Design review of the part shown in the three views and the two pictorial views. Dimensions are in mm from the part's minimum x, y and z. A direction names the side the tool comes from. Give positions to 0.01 mm unless a question says otherwise; leave off trailing zeros. Loops run counter-clockwise (first coordinate to the right, second up) from the corner with the lowest first, then second, coordinate; pieces in that order, holes last.
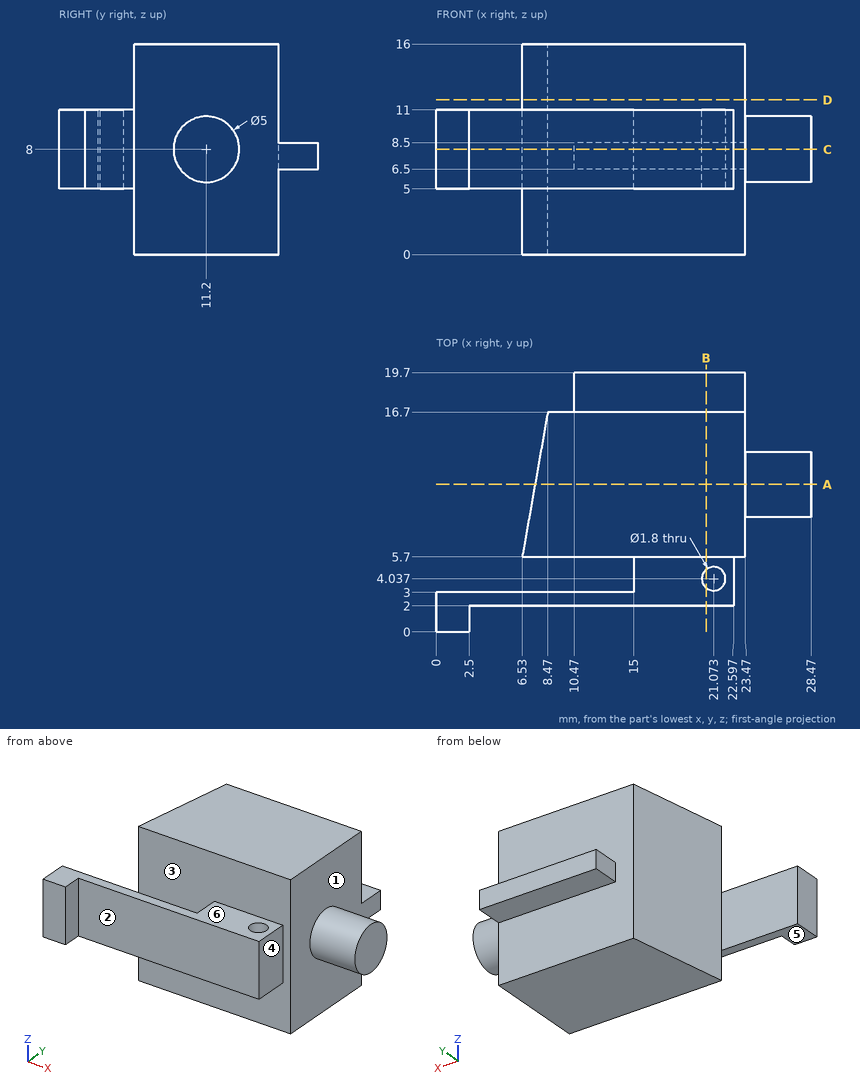
Q1. Consider section A-A on y = 11.2. Give the boundary of the cut face in (x, z).
Answers:
outline: (7.5, 0) - (23.47, 0) - (23.47, 5.5) - (28.47, 5.5) - (28.47, 10.5) - (23.47, 10.5) - (23.47, 16) - (7.5, 16) - close
Q2. Consider section B-B on x = 20.5. Give the boundary of the cut face in (y, z).
Answers:
outline: (2, 5) - (3.34, 5) - (3.34, 11) - (2, 11) - close; (4.73, 5) - (5.7, 5) - (5.7, 0) - (16.7, 0) - (16.7, 6.5) - (19.7, 6.5) - (19.7, 8.5) - (16.7, 8.5) - (16.7, 16) - (5.7, 16) - (5.7, 11) - (4.73, 11) - close
Q3. Mouldability with a two-part tool opening along Y and no side actions: class the marked faces 1, 2 and 3 as +Y half, -Y half, draft (parallel to the pull), parting line (faces both ways), or undercut.
Answers:
face 1: draft
face 2: -Y half
face 3: undercut
Q4. Consider section C-C on z = 8. Give the boundary of the cut face in (x, y), plus the area to 3 significant figures.
Answers:
outline: (0, 0) - (2.5, 0) - (2.5, 2) - (22.6, 2) - (22.6, 5.7) - (23.47, 5.7) - (23.47, 8.7) - (28.47, 8.7) - (28.47, 13.7) - (23.47, 13.7) - (23.47, 19.7) - (10.47, 19.7) - (10.47, 16.7) - (8.47, 16.7) - (6.53, 5.7) - (15, 5.7) - (15, 3) - (0, 3) - close; hole circle Ø1.8 at (21.07, 4.04)
area: 285 mm2
Q5. Machinability: for the marked faces 4, 5 and 6, which of the approach directions +Z, -Z, +X, -X, +Y, -Y give a long, thin tool a straight path to every point of the face, cutting with its end or side? Answer none if there is none.
Answers:
face 4: +Z, -Z, +X, -Y
face 5: -Z, +X, -X, -Y
face 6: +Z, +X, -X, -Y
Q6. For probe 1 along Y at (x, z) = (12.75, 10.25); probe 2 along Y at (x, z) = (14.75, 6.75); probe 3 along Z at (x, y) = (23, 19), list the stretches that pass through material, from the lowest coordinate up.
Answers:
probe 1: y = 2 to 3, 5.7 to 16.7
probe 2: y = 2 to 3, 5.7 to 19.7
probe 3: z = 6.5 to 8.5
Q7. Consider section D-D on z = 11.75. Give the boundary of the cut face in (x, y).
Answers:
outline: (6.53, 5.7) - (23.47, 5.7) - (23.47, 16.7) - (8.47, 16.7) - close
Q8. For pin 1 Ø6.5 at (x, z) = (10, 8) entering from -Y; pin 2 Ø0.6 at (y, z) = (18.5, 7.5) entering from -X; pin 3 Ø1.5 at (x, y) = (14.5, 17.5) entering from -Z, all flat-tipped, find the tip position at first contact; note any pin that passes through.
Answers:
pin 1: stops at y = 2
pin 2: stops at x = 10.47
pin 3: stops at z = 6.5
